```python
from build123d import *
from build123d.topology import SkipClean

# Parameters (mm, degrees)
SKETCH1_R           = 8.5
BOSS_EXTRUDE1_DEPTH = 10
SKETCH2_R           = 8.5
BOSS_EXTRUDE2_DEPTH = 10
SKETCH4_R           = 0.5
SKETCH4_R_2         = 1.5
CUT_EXTRUDE1_DEPTH  = 20
BOSS_EXTRUDE3_DEPTH = 3


with BuildPart() as part:
    # Sketch1 → Boss-Extrude1 (new body)
    with BuildSketch(Plane.XY):
        Circle(SKETCH1_R)
    extrude(amount=BOSS_EXTRUDE1_DEPTH)

    # Sketch2 → Boss-Extrude2 (add)
    with BuildSketch(Plane.XY.offset(10)):
        with Locations(Location((0, -1.5, 0), (0, 0, 174.937907036))):
            Circle(SKETCH2_R)
    extrude(amount=BOSS_EXTRUDE2_DEPTH)

    # Sketch4 → Cut-Extrude1 (cut)
    with BuildSketch(Plane.XY.offset(20)):
        Circle(SKETCH4_R)
        with Locations((-5, 0)):
            Circle(SKETCH4_R_2)
        with Locations((5, 0)):
            Circle(SKETCH4_R_2)
    extrude(amount=-CUT_EXTRUDE1_DEPTH, mode=Mode.SUBTRACT)

    # Sketch5 → Boss-Extrude3 (add)
    with SkipClean():  # the faces are left unmerged after this step: merging them gives an invalid solid
        with BuildSketch(Plane.XY.offset(20)):
            with BuildLine():
                ThreePointArc((-8.366600265, 0), (0, -7), (8.366600265, 0))
                ThreePointArc((8.366600265, 0), (0, -10), (-8.366600265, 0))
            make_face()
        extrude(amount=BOSS_EXTRUDE3_DEPTH)


solid = part.part
```
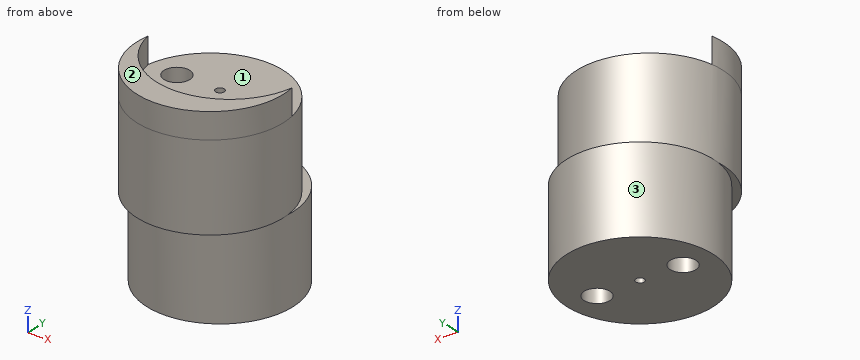
The listing builds one solid part. Answer for the finished solid, in the listing's coordinates (mm). Face numbers are marked on the shaded views. Give positions to 0.01 mm unless a question says otherwise; leave off trailing zeros. Order: outer loops, then holes, each group sorted by start corner. A loop starts at its lowest first (then second) coordinate and runs counter-clockwise, first axis right, second up. Notation, with made-up numbers: (63.25, 6) -> (83.25, 6) arc R26 ccw to (83.25, 23) -> close; hole circle Ø9 at (0, -4.5). An arc over 180 degrees is marked (long way). Answer as a JSON object with one key per item and string values. Group by question number.
Item 1: Consider L1, parallel to Y at x = 0, z = 2.75; L2, parallel to Y at x = 0, z = 12.5; L3, parallel to X at y = 0.75, z = 7.5. Determine where each line is inside the solid, lowest interval first. Write a range as from..to.
Item 2: Flat-ended cylindrical pins translate along their axes: pin 1 (1 mm diameter, centred on x = -3.5, z = 4, fed in from -Y); pin 2 (5 mm diameter, centred on x = -1.5, y = 1, fed in from +Z); pin 3 (3 mm diameter, centred on y = -6.5, z = 4, fed in from +X). Find the tip coordinate at first contact, or state that the pin passes through.
Item 3: The part is cut by section D-D on z = 19. Write down the section's boundary in (x, y).
Item 4: Determine the mould class of the marked faces 1, 2 and 3 for opening direction X: pulls with the +X half, pulls with the -X half, needs draft (parallel to the pull), parting line crosses it, or undercut.
Item 5: The part is cut by section A-A on x = 0. Write down the section's boundary in (y, z), and give its area (3 significant figures).
Item 6: The part is cut by section B-B on y = 3.75. Write down the section's boundary in (x, z), and give its area (3 significant figures).
Item 7: The part is cut by section C-C on x = 4.5. Write down the section's boundary in (y, z), and give its area (3 significant figures).
Result set:
{
 "1": {"L1": "-8.5..-0.5, 0.5..8.5", "L2": "-10..-0.5, 0.5..7", "L3": "-8.47..-6.3, -3.7..3.7, 6.3..8.47"},
 "2": {"pin 1": "y = -7.95", "pin 2": "z = 20", "pin 3": "x = 6.87"},
 "3": {"outline": "circle Ø17 at (0, -1.5); hole circle Ø3 at (-5, 0); hole circle Ø1 at (0, 0); hole circle Ø3 at (5, 0)"},
 "4": {"face 1": "undercut", "face 2": "needs draft", "face 3": "parting line crosses it"},
 "5": {"outline": "(-10, 10) -> (-8.5, 10) -> (-8.5, 0) -> (-0.5, 0) -> (-0.5, 20) -> (-7, 20) -> (-7, 23) -> (-10, 23) -> close; (0.5, 0) -> (8.5, 0) -> (8.5, 10) -> (7, 10) -> (7, 20) -> (0.5, 20) -> close", "area": "329 mm²"},
 "6": {"outline": "(-7.63, 0) -> (7.63, 0) -> (7.63, 10) -> (6.68, 10) -> (6.68, 20) -> (-6.68, 20) -> (-6.68, 10) -> (-7.63, 10) -> close", "area": "286 mm²"},
 "7": {"outline": "(-8.71, 10) -> (-7.21, 10) -> (-7.21, 0) -> (-1.41, 0) -> (-1.41, 20) -> (-5.71, 20) -> (-5.71, 23) -> (-8.71, 23) -> close; (1.41, 0) -> (7.21, 0) -> (7.21, 10) -> (5.71, 10) -> (5.71, 20) -> (1.41, 20) -> close", "area": "241 mm²"}
}
